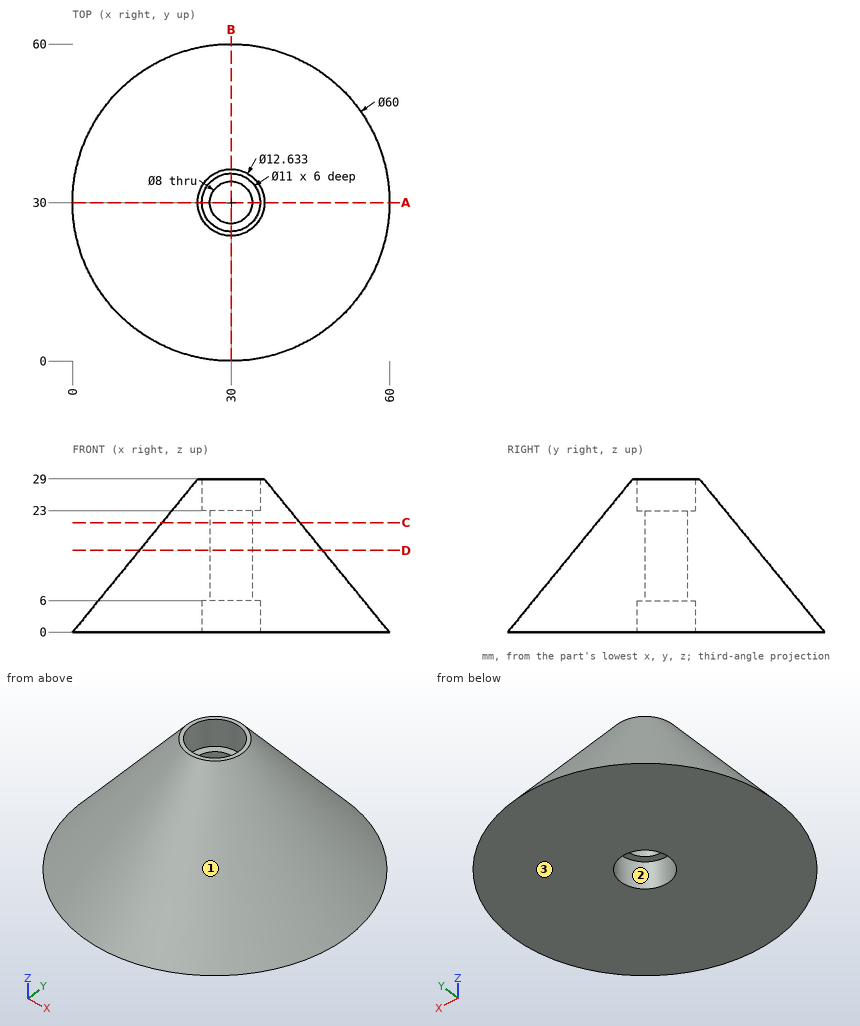
The drawing under review shows one solid part. Ordinate dimensions are in mm from its lowest x, y, z. Give positions to 0.01 mm unless a question says otherwise; leave off trailing zeros. Order: outer loops, then holes, each group sorted by start corner. A loop starts at its lowest first (then second) coordinate and runs counter-clockwise, first axis right, second up. Notation, with made-up numbers: (41, 63) -> (59, 63) arc R22 ccw to (59, 101) -> close; hole circle Ø4 at (24.25, -38.75). An arc over 180 degrees is marked (long way). Write item = value, one per line. Start each with the question number.
(1) We need section D-D on z = 15.5. Write out the cut boundary in (x, y).
(2) We need section C-C on z = 20.75. Write out the cut boundary in (x, y) (1 decimal), plus the area to 3 significant figures.
(3) We need section A-A on y = 30. Write out the cut boundary in (x, z).
(4) To check wall thickness, follow line 1 along Y through (x, z) = (30, 13) (1 decimal); line 2 along X through (y, z) = (26, 3.75) (1 decimal); line 3 along Y through (x, z) = (30, 9). State the ranges of each line that lie inside material, in increasing order.
(5) For pin 1 (12 mm diameter, centred on y = 34, z = 21.5, fed in from +X) (1 decimal); pin 2 (4 mm diameter, centred on x = 35.5, z = 23, fed in from +Y); pin 3 (12 mm diameter, centred on x = 42, z = 21.5, fed in from -Y); pin 4 (6.5 mm diameter, centred on x = 30, y = 30, fed in from +Z), all flat-tipped, find the tip position at first contact; note any pin that passes through.
(6) Mouldability with a two-part tool opening along Y and no side actions: class the marked faces 1, 2 and 3 as +Y half, -Y half, draft (parallel to the pull), parting line (faces both ways), or undercut.
Numbers:
q1.outline = circle Ø34.68 at (30, 30); hole circle Ø8 at (30, 30)
q2.outline = circle Ø26.1 at (30, 30); hole circle Ø8 at (30, 30)
q2.area = 485 mm^2
q3.outline = (0, 0) -> (24.5, 0) -> (24.5, 6) -> (26, 6) -> (26, 23) -> (24.5, 23) -> (24.5, 29) -> (23.68, 29) -> close; (34, 6) -> (35.5, 6) -> (35.5, 0) -> (60, 0) -> (36.32, 29) -> (35.5, 29) -> (35.5, 23) -> (34, 23) -> close
q4.line_1 = 10.6 to 26, 34 to 49.4
q4.line_2 = 3.4 to 26.2, 33.8 to 56.6
q4.line_3 = 7.35 to 26, 34 to 52.65
q5.pin_1 = 47
q5.pin_2 = 41.81
q5.pin_3 = 15.94
q5.pin_4 = through
q6.face_1 = parting line
q6.face_2 = undercut
q6.face_3 = draft
